Source: three-view drawing plus pictorial views. Frame: mm from the lowest corner of the part. A direction names the side the tool comes from. Round coordinates to 2 decimals unless told otherwise and drop trailing zeros. Write each loop counter-clockwise with the first axis right and the second up, starting at its lowest first coordinate (ties: lowest second). Pieces come first, ordered by that corner, then holes. Notation, with made-up numbers: (76.5, 73.25) -> (99.5, 73.25) arc R31 cw to (99.5, 98.25) -> close; hole circle Ø2 at (65, 49). An arc over 180 degrees is marked (long way). Put each result on its own line as item: value.
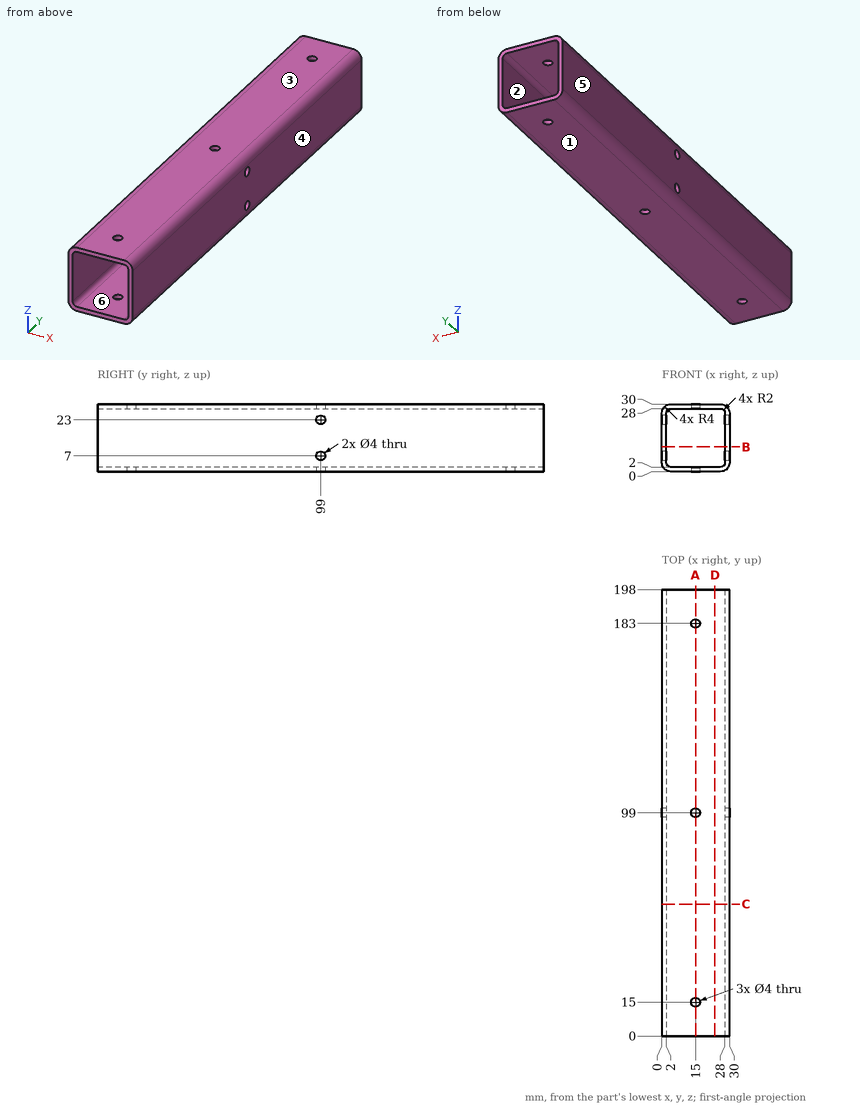
Q1. Material intervals for line 1 (Y direction, x = 15, z = 28.9); line 2 (X direction, y = 185.5, z = 26), sorted ascending. Write a range as [from, to].
Ans:
line 1: y = [0, 13], [17, 97], [101, 181], [185, 198]
line 2: x = [0, 2], [28, 30]
Q2. Cut plane D-D on x = 23.5. Output: boundary loops of the cut face in (y, z).
Ans:
outline: (0, 0) -> (198, 0) -> (198, 2) -> (0, 2) -> close; (0, 28) -> (198, 28) -> (198, 30) -> (0, 30) -> close
Q3. Draft query along X for the marked faces 3, 4, 5 and 6. Return one class per face: +X half, -X half, draft (parallel to the pull), parting line (faces both ways), or undercut.
Ans:
face 3: draft
face 4: +X half
face 5: -X half
face 6: undercut
Q4. Cut plane A-A on x = 15. Give the number of separate pieces and of enclosed holes in the cut face, and give its area (3 significant figures).
Ans:
separate pieces: 8
enclosed holes: 0
area: 744 mm^2
Q5. Reachability of the marked faces 1 and 2 from +Z, -Z, +X, -X, +Y, -Y: full face, straight path, thin tool, end or side. Return the list, or none.
Ans:
face 1: -Z, +X, -X, +Y, -Y
face 2: +Y, -Y
Q6. Cut plane C-C on y = 58.5. Output: boundary loops of the cut face in (x, z), and give its area (3 significant figures).
Ans:
outline: (0, 4) arc R4 ccw to (4, 0) -> (26, 0) arc R4 ccw to (30, 4) -> (30, 26) arc R4 ccw to (26, 30) -> (4, 30) arc R4 ccw to (0, 26) -> close; hole (2, 4) arc R2 ccw to (4, 2) -> (26, 2) arc R2 ccw to (28, 4) -> (28, 26) arc R2 ccw to (26, 28) -> (4, 28) arc R2 ccw to (2, 26) -> close
area: 214 mm^2
Q7. Cut plane B-B on z = 11. Output: boundary loops of the cut face in (x, y).
Ans:
outline: (0, 0) -> (2, 0) -> (2, 198) -> (0, 198) -> close; (28, 0) -> (30, 0) -> (30, 198) -> (28, 198) -> close
